Geometry: final body of the model. Coordinates: model frame, mm. Face numbers are marked on the shaded views. Give positions to 0.01 mm unless a question says otherwise; leave off trailing zeros. Write each loop counter-clockwise with the first axis right and the second up, starting at its lowest first coordinate (ties: lowest second). Pieces come first, ordered by that corner, then holes. Notation, with made-up numbers: (70, -4.75) -> (75, -4.75) arc R17 ccw to (75, 11.25) -> close; hole circle Ø9 at (26, -9). An arc over 180 degrees is marked (long way). Answer as a JSON object with one key per item and string values. Group by question number.
(1) Section query D-D on x = 33.5. Output: boundary loops of the cut face in (y, z), plus the area to 3 significant figures.
(2) Section query B-B on z = 1.25. State how many separate pieces and enclosed holes the cut face has, plus the area to 3 significant figures.
(3) Section query A-A on y = 7. Output: boundary loops of the cut face in (x, z) (3 decimals), plus the area to 3 significant figures.
(4) Draft query along X for the marked faces 1, 2, 3 and 4. Return one class per face: +X half, -X half, draft (parallel to the pull), parting line (faces both ways), or undercut.
(5) Material intervals for probe 1 along Y at (x, z) = (0, 3.65); probe 2 along Y at (x, z) = (0, 1.35) (3 decimals); probe 3 along X at (y, z) = (26.5, -0.5), sorted ascending.
(6) Contact query for flat-ended pins moving along their axis: pin 1 Ø2.5 at (x, y) = (-4.79, 35.16) entering from -Z; pin 2 Ø3.5 at (x, y) = (-12.99, 29.5) entering from -Z; pin 3 Ø5 at (x, y) = (12.99, 29.5) entering from +Z. Output: stop coordinate, or through.
(7) Section query C-C on x = 0. Output: boundary loops of the cut face in (y, z) (3 decimals), plus the area to 3 significant figures.
from build123d import *

# Parameters (mm, degrees)
ESQUISSE3_R                  = 3.5
BOSS_EXTRU_1_DEPTH           = 44
ESQUISSE4_R                  = 10.25
ESQUISSE4_R_2                = 1.625
ENL_V_MAT_EXTRU_1_DEPTH      = 60
ENL_V_MAT_EXTRU_2_DEPTH      = 60.816385715
ENL_V_MAT_EXTRU_2_DEPTH_BACK = 3
ESQUISSE6_R                  = 3.1


with BuildPart() as part:
    # Esquisse3 → Boss.-Extru.1 (new body)
    with BuildSketch(Plane(origin=(0, 0, 0), x_dir=(1, 0, 0), z_dir=(0, 1, 0))):
        with BuildLine():
            Line((26, 0), (-26, 0))
            ThreePointArc((-26, 0), (-27.414213562, 0.585786438), (-28, 2))
            Line((-28, 2), (-28, 4))
            ThreePointArc((-28, 4), (-28.585786438, 5.414213562), (-30, 6))
            Line((-30, 6), (-37, 6))
            ThreePointArc((-37, 6), (-38.414213562, 5.414213562), (-39, 4))
            Line((-39, 4), (-39, -3))
            ThreePointArc((-39, -3), (-38.414213562, -4.414213562), (-37, -5))
            Line((-37, -5), (37, -5))
            ThreePointArc((37, -5), (38.414213562, -4.414213562), (39, -3))
            Line((39, -3), (39, 4))
            ThreePointArc((39, 4), (38.414213562, 5.414213562), (37, 6))
            Line((37, 6), (30, 6))
            ThreePointArc((30, 6), (28.585786438, 5.414213562), (28, 4))
            Line((28, 4), (28, 2))
            ThreePointArc((28, 2), (27.414213562, 0.585786438), (26, 0))
        make_face()
        with Locations(Location((-33.5, 0.5, 0), (0, 0, 270))):
            Circle(ESQUISSE3_R, mode=Mode.SUBTRACT)
        with Locations(Location((33.5, 0.5, 0), (0, 0, 90))):
            Circle(ESQUISSE3_R, mode=Mode.SUBTRACT)
    extrude(amount=BOSS_EXTRU_1_DEPTH)

    # Esquisse4 → Enlèv. mat.-Extru.1 (cut)
    with BuildSketch(Plane.XY.offset(5)):
        with Locations((0, 22)):
            Circle(ESQUISSE4_R)
        with Locations((0, 7)):
            Circle(ESQUISSE4_R_2)
        with Locations((-8.999026536, 11.275377796)):
            Circle(ESQUISSE4_R_2)
        with Locations((13.787308542, 19.568925513)):
            Circle(ESQUISSE4_R_2)
        with Locations((12.990381057, 29.5)):
            Circle(ESQUISSE4_R_2)
        with Locations((-4.788282007, 35.155696691)):
            Circle(ESQUISSE4_R_2)
        with Locations((-12.990381057, 29.5)):
            Circle(ESQUISSE4_R_2)
    extrude(amount=-ENL_V_MAT_EXTRU_1_DEPTH, mode=Mode.SUBTRACT)

    # Esquisse6 → Enlèv. mat.-Extru.2 (cut, two sides: drawn at the far end of the back side and taken through both)
    with BuildSketch(Plane.XY.offset(5).offset(-ENL_V_MAT_EXTRU_2_DEPTH_BACK)):
        with Locations(Location((0, 7, 0), (0, 0, 180))):
            Circle(ESQUISSE6_R)
        with Locations(Location((-8.999026536, 11.275377796, 0), (0, 0, 180))):
            Circle(ESQUISSE6_R)
        with Locations(Location((-4.788282007, 35.155696691, 0), (0, 0, 180))):
            Circle(ESQUISSE6_R)
        with Locations(Location((-12.990381057, 29.5, 0), (0, 0, 180))):
            Circle(ESQUISSE6_R)
        with Locations(Location((13.787308542, 19.568925513, 0), (0, 0, 180))):
            Circle(ESQUISSE6_R)
        with Locations(Location((12.990381057, 29.5, 0), (0, 0, 180))):
            Circle(ESQUISSE6_R)
    extrude(amount=ENL_V_MAT_EXTRU_2_DEPTH + ENL_V_MAT_EXTRU_2_DEPTH_BACK, mode=Mode.SUBTRACT)


solid = part.part
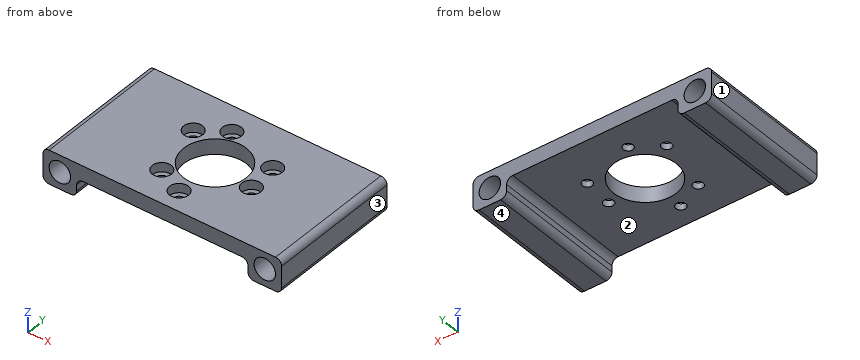
Answer list:
{
 "1": {"outline": "(0, -6) -> (44, -6) -> (44, -4) -> (0, -4) -> close; (0, 3) -> (44, 3) -> (44, 5) -> (0, 5) -> close", "area": "176 mm2"},
 "2": {"separate pieces": "3", "enclosed holes": "7", "area": "2,520 mm2"},
 "3": {"outline": "(-39, -4) arc R2 ccw to (-37, -6) -> (-30, -6) arc R2 ccw to (-28, -4) -> (-28, -2) arc R2 cw to (-26, 0) -> (-1.625, 0) -> (-1.625, 2) -> (-3.1, 2) -> (-3.1, 5) -> (-37, 5) arc R2 ccw to (-39, 3) -> close; (1.625, 0) -> (26, 0) arc R2 cw to (28, -2) -> (28, -4) arc R2 ccw to (30, -6) -> (37, -6) arc R2 ccw to (39, -4) -> (39, 3) arc R2 ccw to (37, 5) -> (3.1, 5) -> (3.1, 2) -> (1.625, 2) -> close; hole circle Ø7 at (-33.5, -0.5); hole circle Ø7 at (33.5, -0.5)", "area": "416 mm2"},
 "4": {"face 1": "-X half", "face 2": "undercut", "face 3": "+X half", "face 4": "draft"},
 "5": {"probe 1": "0 to 3.9, 10.1 to 11.75, 32.25 to 44", "probe 2": "0 to 5.375, 8.625 to 11.75, 32.25 to 44", "probe 3": "-39 to -37, -30 to -27.32, 27.32 to 30, 37 to 39"},
 "6": {"pin 1": "through", "pin 2": "z = 0", "pin 3": "z = 2"},
 "7": {"outline": "(0, 0) -> (5.375, 0) -> (5.375, 2) -> (3.9, 2) -> (3.9, 5) -> (0, 5) -> close; (8.625, 0) -> (11.75, 0) -> (11.75, 5) -> (10.1, 5) -> (10.1, 2) -> (8.625, 2) -> close; (32.25, 0) -> (44, 0) -> (44, 5) -> (32.25, 5) -> close", "area": "92.4 mm2"}
}
